from build123d import *

# Parameters (mm, degrees)
F1_DEPTH = 12
F2_T     = -2.5


with BuildPart() as f1:
    # F0 (on Top) → F1 (new body)
    with BuildSketch(Plane.XY):
        with BuildLine():
            ThreePointArc((5, 12), (1.464466, 10.535534), (0, 7))
            Line((0, 7), (0, 0))
            Line((0, 0), (0, -7))
            ThreePointArc((0, -7), (1.464466, -10.535534), (5, -12))
            Line((5, -12), (17.113249, -12))
            ThreePointArc((17.113249, -12), (19.613249, -11.330127), (21.443376, -9.5))
            Line((21.443376, -9.5), (25.484828, -2.5))
            ThreePointArc((25.484828, -2.5), (26.154701, 0), (25.484828, 2.5))
            Line((25.484828, 2.5), (21.443376, 9.5))
            ThreePointArc((21.443376, 9.5), (19.613249, 11.330127), (17.113249, 12))
            Line((17.113249, 12), (5, 12))
        make_face()
    extrude(amount=F1_DEPTH)

    # F2
    f2_openings = [f1.faces().sort_by_distance(p)[0] for p in [
        (11.952499, 0, 12),
    ]]
    offset(amount=F2_T, openings=f2_openings)


solid = f1.part
The model under review builds one solid part; all positions refer to its coordinate system, in mm. A direction names the side the tool comes from. Coordinates: 2 decimals unless noted, no trailing zeros. Loops run counter-clockwise (first coordinate to the right, second up) from the corner with the lowest first, then second, coordinate; pieces in that order, holes last. Notation, with made-up numbers: (-0.5, -39) -> (44.5, -39) arc R30 ccw to (44.5, -5) -> close; hole circle Ø3 at (57.25, 52). An arc over 180 degrees is marked (long way). Use a Markdown table: item, result. Add a question column.
1. Clearance check with flat-ended pins moving along their axes: pin 1 Ø5 at (x, y) = (15.5, 1) entering from +Z; pin 2 Ø4 at (y, z) = (-4, 4.5) entering from +X; pin 3 Ø3 at (y, z) = (-9, 9) entering from +X. State where each tip first meets the part, or that it passes through.
2. To check wall thickness, follow line 1 (Y direction, x = 8, z = 4); line 2 (Z direction, x = 18.75, y = 7.5); line 3 (X direction, y = -7.25, z = 8.5). State the ranges of each line that lie inside material, in increasing order.
3. Add section C-C on z = 2. Write out the cut boundary in (x, y).
4. Add section D-D on y = 0.5. Write out the cut boundary in (x, z), plus the area to 3 significant figures.
5. Draft analysis for pull direction Y (two halves, no side actions). For faces 3 (the face through (2, 11, 6)), 4 (the face through (21.27, -4.8, 7.18)), 5 (the face through (19.58, -11.35, 5.92)), state which applies: pulls with the +Y half, pulls with the -Y half, needs draft (parallel to the pull), parting line crosses it, or undercut.
6. Add section A-A on z = 11.25. Write out the cut boundary in (x, y).
7. Add section B-B on x = 15.75. Write out the cut boundary in (y, z).
8. Machinability: for faces 1 (the face through (23.655, -0.018, 7.184)), 2 (the face through (26.155, -0.037, 5.916)), which of the approach directions +Z, -Z, +X, -X, +Y, -Y give a long, thin tool a straight path to every point of the face, cutting with its end or side? Answer none if there is none.
Returned:
| question | item | result |
|---|---|---|
| 1 | pin 1 | stops at z = 2.5 |
| 1 | pin 2 | stops at x = 25.74 |
| 1 | pin 3 | stops at x = 22.6 |
| 2 | line 1 | y = -12 to -9.5, 9.5 to 12 |
| 2 | line 2 | z = 0 to 2.5 |
| 2 | line 3 | x = 0.01 to 2.51, 19.86 to 22.74 |
| 3 | outline | (0, -7) arc R5 ccw to (5, -12) -> (17.11, -12) arc R5 ccw to (21.44, -9.5) -> (25.48, -2.5) arc R5 ccw to (25.48, 2.5) -> (21.44, 9.5) arc R5 ccw to (17.11, 12) -> (5, 12) arc R5 ccw to (0, 7) -> close |
| 4 | outline | (0, 0) -> (26.13, 0) -> (26.13, 12) -> (23.6, 12) -> (23.6, 2.5) -> (2.5, 2.5) -> (2.5, 12) -> (0, 12) -> close |
| 4 | area | 113 mm² |
| 5 | face 3 | pulls with the +Y half |
| 5 | face 4 | undercut |
| 5 | face 5 | pulls with the -Y half |
| 6 | outline | (0, -7) arc R5 ccw to (5, -12) -> (17.11, -12) arc R5 ccw to (21.44, -9.5) -> (25.48, -2.5) arc R5 ccw to (25.48, 2.5) -> (21.44, 9.5) arc R5 ccw to (17.11, 12) -> (5, 12) arc R5 ccw to (0, 7) -> close; hole (2.5, -7) arc R2.5 ccw to (5, -9.5) -> (17.11, -9.5) arc R2.5 ccw to (19.28, -8.25) -> (23.32, -1.25) arc R2.5 ccw to (23.32, 1.25) -> (19.28, 8.25) arc R2.5 ccw to (17.11, 9.5) -> (5, 9.5) arc R2.5 ccw to (2.5, 7) -> close |
| 7 | outline | (-12, 0) -> (12, 0) -> (12, 12) -> (9.5, 12) -> (9.5, 2.5) -> (-9.5, 2.5) -> (-9.5, 12) -> (-12, 12) -> close |
| 8 | face 1 | +Z |
| 8 | face 2 | +Z, -Z, +X |
